Model file for the job. Use its own axes, mm. A direction names the side the tool comes from. Give positions to 0.01 mm unless a question says otherwise; leave off trailing zeros. Loops run counter-clockwise (first coordinate to the right, second up) from the corner with the lowest first, then second, coordinate; pieces in that order, holes last. Notation, with made-up numbers: M -27.75,-7 L 0.25,-7 A21 cw 0.25,18 Z; hole C 33,-40 d9. An arc over 180 degrees is marked long. Answer in a Markdown table with one row per item.
```python
from build123d import *

# Parameters (mm, degrees)
BOSS_EXTRUDE1_DEPTH     = 13
SKETCH6_W               = 6
SKETCH6_H               = 5
BOSS_EXTRUDE4_DEPTH     = 5.6
SKETCH16_W              = 6
SKETCH16_H              = 8
BOSS_EXTRUDE5_DEPTH     = 0.1
CUT_EXTRUDE6_DEPTH      = 4
CUT_EXTRUDE6_DEPTH_BACK = 3.6
SKETCH15_R              = 1.2
CUT_EXTRUDE7_DEPTH      = 8.7202
CUT_EXTRUDE8_START      = -0.2202
SKETCH19_W              = 6
SKETCH19_H              = 8
SKETCH19_R              = 1.2
CUT_EXTRUDE8_DEPTH      = 0.2202
SKETCH12_R              = 1.5
CUT_EXTRUDE5_DEPTH      = 6
CHAMFER1_SIZE           = 0.2
SKETCH20_W              = 5
SKETCH20_H              = 5.5
BOSS_EXTRUDE6_DEPTH     = 0.5
SKETCH21_W              = 5
SKETCH21_H              = 5.5
BOSS_EXTRUDE7_DEPTH     = 0.5
CHAMFER2_SIZE           = 0.2


with BuildPart() as part:
    # Sketch1 → Boss-Extrude1 (new body)
    with BuildSketch(Plane.XY):
        Polygon((3, 3.05), (3, -2.253801214), (2.388188946, -2.95), (-2.388188946, -2.95), (-3, -2.253801214), (-3, 3.05), align=None)
    extrude(amount=BOSS_EXTRUDE1_DEPTH)

    # Sketch6 → Boss-Extrude4 (add)
    with BuildSketch(Plane(origin=(0, 3.05, 0), x_dir=(1, 0, 0), z_dir=(0, 1, 0))):
        with Locations((0, -2.5)):
            Rectangle(SKETCH6_W, SKETCH6_H)
    extrude(amount=BOSS_EXTRUDE4_DEPTH)

    # Sketch16 → Boss-Extrude5 (add)
    with BuildSketch(Plane(origin=(0, 3.05, 0), x_dir=(1, 0, 0), z_dir=(0, 1, 0))):
        with Locations((0, -9)):
            Rectangle(SKETCH16_W, SKETCH16_H)
    extrude(amount=BOSS_EXTRUDE5_DEPTH)

    # Sketch18 → Cut-Extrude6 (cut, two sides: drawn at the far end of the back side and taken through both)
    with BuildSketch(Plane(origin=(0, 0, 0), x_dir=(0, 0, -1), z_dir=(1, 0, 0)).offset(-CUT_EXTRUDE6_DEPTH_BACK)):
        with BuildLine():
            Line((-8.8572, -0.0702), (-12.8572, -0.0702))
            Line((-12.8572, -0.0702), (-13, -0.0702))
            Line((-13, -0.0702), (-13, -0.7))
            Line((-13, -0.7), (-12.8572, -0.7))
            Line((-12.8572, -0.7), (-12.7144, -0.7))
            add(Edge.make_bspline(
                [(-12.7144, -0.7), (-12.5198, -0.7), (-12.43, -0.9509)],
                knots=[0.103448276, 0.103448276, 0.103448276, 0.137931034, 0.137931034, 0.137931034], degree=2))
            add(Edge.make_bspline(
                [(-12.43, -0.9509), (-12.3594, -1.2388), (-12.13, -1.45), (-11.8572, -1.45)],
                knots=[0.137931034, 0.137931034, 0.137931034, 0.137931034, 0.172413793, 0.172413793, 0.172413793, 0.172413793], degree=3))
            add(Edge.make_bspline(
                [(-11.8572, -1.45), (-11.5844, -1.45), (-11.355, -1.2388), (-11.2844, -0.9509)],
                knots=[0.172413793, 0.172413793, 0.172413793, 0.172413793, 0.206896552, 0.206896552, 0.206896552, 0.206896552], degree=3))
            add(Edge.make_bspline(
                [(-11.2844, -0.9509), (-11.1946, -0.7), (-11, -0.7)],
                knots=[0.206896552, 0.206896552, 0.206896552, 0.24137931, 0.24137931, 0.24137931], degree=2))
            Line((-11, -0.7), (-10.8572, -0.7))
            Line((-10.8572, -0.7), (-10.7144, -0.7))
            add(Edge.make_bspline(
                [(-10.7144, -0.7), (-10.5198, -0.7), (-10.43, -0.9509)],
                knots=[0.310344828, 0.310344828, 0.310344828, 0.344827586, 0.344827586, 0.344827586], degree=2))
            add(Edge.make_bspline(
                [(-10.43, -0.9509), (-10.3594, -1.2388), (-10.13, -1.45), (-9.8572, -1.45)],
                knots=[0.344827586, 0.344827586, 0.344827586, 0.344827586, 0.379310345, 0.379310345, 0.379310345, 0.379310345], degree=3))
            add(Edge.make_bspline(
                [(-9.8572, -1.45), (-9.5844, -1.45), (-9.355, -1.2388), (-9.2844, -0.9509)],
                knots=[0.379310345, 0.379310345, 0.379310345, 0.379310345, 0.413793103, 0.413793103, 0.413793103, 0.413793103], degree=3))
            add(Edge.make_bspline(
                [(-9.2844, -0.9509), (-9.1946, -0.7), (-9, -0.7)],
                knots=[0.413793103, 0.413793103, 0.413793103, 0.448275862, 0.448275862, 0.448275862], degree=2))
            Line((-9, -0.7), (-8.8572, -0.7))
            Line((-8.8572, -0.7), (-8.7144, -0.7))
            add(Edge.make_bspline(
                [(-8.7144, -0.7), (-8.5198, -0.7), (-8.43, -0.9509)],
                knots=[0.517241379, 0.517241379, 0.517241379, 0.551724138, 0.551724138, 0.551724138], degree=2))
            add(Edge.make_bspline(
                [(-8.43, -0.9509), (-8.3594, -1.2388), (-8.13, -1.45), (-7.8572, -1.45)],
                knots=[0.551724138, 0.551724138, 0.551724138, 0.551724138, 0.586206897, 0.586206897, 0.586206897, 0.586206897], degree=3))
            add(Edge.make_bspline(
                [(-7.8572, -1.45), (-7.5844, -1.45), (-7.355, -1.2388), (-7.2844, -0.9509)],
                knots=[0.586206897, 0.586206897, 0.586206897, 0.586206897, 0.620689655, 0.620689655, 0.620689655, 0.620689655], degree=3))
            add(Edge.make_bspline(
                [(-7.2844, -0.9509), (-7.1946, -0.7), (-7, -0.7)],
                knots=[0.620689655, 0.620689655, 0.620689655, 0.655172414, 0.655172414, 0.655172414], degree=2))
            Line((-7, -0.7), (-6.8572, -0.7))
            Line((-6.8572, -0.7), (-6.7144, -0.7))
            add(Edge.make_bspline(
                [(-6.7144, -0.7), (-6.5198, -0.7), (-6.43, -0.9509)],
                knots=[0.724137931, 0.724137931, 0.724137931, 0.75862069, 0.75862069, 0.75862069], degree=2))
            add(Edge.make_bspline(
                [(-6.43, -0.9509), (-6.3594, -1.2388), (-6.13, -1.45), (-5.8572, -1.45)],
                knots=[0.75862069, 0.75862069, 0.75862069, 0.75862069, 0.793103448, 0.793103448, 0.793103448, 0.793103448], degree=3))
            add(Edge.make_bspline(
                [(-5.8572, -1.45), (-5.5844, -1.45), (-5.355, -1.2388), (-5.2844, -0.9509)],
                knots=[0.793103448, 0.793103448, 0.793103448, 0.793103448, 0.827586207, 0.827586207, 0.827586207, 0.827586207], degree=3))
            add(Edge.make_bspline(
                [(-5.2844, -0.9509), (-5.1946, -0.7), (-5, -0.7)],
                knots=[0.827586207, 0.827586207, 0.827586207, 0.862068966, 0.862068966, 0.862068966], degree=2))
            Line((-5, -0.7), (-5, -0.0702))
            Line((-5, -0.0702), (-8.8572, -0.0702))
        make_face()
    extrude(amount=CUT_EXTRUDE6_DEPTH + CUT_EXTRUDE6_DEPTH_BACK, mode=Mode.SUBTRACT)

    # Sketch15 → Cut-Extrude7 (cut)
    with BuildSketch(Plane(origin=(0, 8.65, 0), x_dir=(1, 0, 0), z_dir=(0, 1, 0))):
        with Locations(Location((0, -10.8572, 0), (0, 0, 180))):
            Circle(SKETCH15_R)
        with Locations(Location((0, -6.8572, 0), (0, 0, 180))):
            Circle(SKETCH15_R)
    extrude(amount=-CUT_EXTRUDE7_DEPTH, mode=Mode.SUBTRACT)

    # Sketch19 → Cut-Extrude8 (cut)
    with BuildSketch(Plane.XZ.offset(0.0702).offset(CUT_EXTRUDE8_START)):
        with Locations((0, 9)):
            Rectangle(SKETCH19_W, SKETCH19_H)
        with Locations(Location((0, 10.8572, 0), (0, 0, 180))):
            Circle(SKETCH19_R, mode=Mode.SUBTRACT)
        with Locations(Location((0, 6.8572, 0), (0, 0, 180))):
            Circle(SKETCH19_R, mode=Mode.SUBTRACT)
    extrude(amount=CUT_EXTRUDE8_DEPTH, mode=Mode.SUBTRACT)

    # Sketch12 → Cut-Extrude5 (cut)
    with BuildSketch(Plane.XY.offset(5)):
        with Locations((0, 5.9)):
            Circle(SKETCH12_R)
    extrude(amount=-CUT_EXTRUDE5_DEPTH, mode=Mode.SUBTRACT)

    # Chamfer1
    chamfer1_edges = [part.edges().sort_by_distance(p)[0] for p in [
        (-2.694094473, -2.601900607, 13),
        (0, -2.95, 13),
        (2.694094473, -2.601900607, 13),
        (3, 1.65, 13),
        (3, -1.476900607, 13),
        (-3, -1.476900607, 13),
        (-3, 1.65, 13),
    ]]
    chamfer(chamfer1_edges, length=CHAMFER1_SIZE)

    # Sketch20 → Boss-Extrude6 (add)
    with BuildSketch(Plane(origin=(3, 0, 0), x_dir=(0, 0, -1), z_dir=(1, 0, 0))):
        with Locations((-2.5, 5.9)):
            Rectangle(SKETCH20_W, SKETCH20_H)
    extrude(amount=BOSS_EXTRUDE6_DEPTH)

    # Sketch21 → Boss-Extrude7 (add)
    with BuildSketch(Plane.ZY.offset(3)):
        with Locations((2.5, 5.9)):
            Rectangle(SKETCH21_W, SKETCH21_H)
    extrude(amount=BOSS_EXTRUDE7_DEPTH)

    # Chamfer2
    chamfer2_edges = [part.edges().sort_by_distance(p)[0] for p in [
        (3.5, 5.9, 5),
        (-3.5, 5.9, 5),
    ]]
    chamfer(chamfer2_edges, length=CHAMFER2_SIZE)


solid = part.part
```
(1) Mould opens along Y. For faces 4 (the flat face through (0, 8.65, 2)), 5 (the flat face through (-3, 0.4, 6.5)), 6 (the flat face through (0, -2.95, 6)), 7 (the cylindrical face through (-0.195, 7.387, 2.535)) say: pulls with the +Y half, pulls with the -Y half, needs draft (parallel to the pull), parting line crosses it, or undercut.
Established:
| item | result |
|---|---|
| face 4 | pulls with the +Y half |
| face 5 | needs draft |
| face 6 | pulls with the -Y half |
| face 7 | undercut |
(2) Saw through at C-C, the plane x = 0. Count the separate pieces of the cut face and the enclosed holes in it, and give its area (3 significant figures).
Established:
| item | result |
|---|---|
| separate pieces | 4 |
| enclosed holes | 0 |
| area | 67.6 mm2 |
(3) Flat gauge pins, fed straight in: P1, Ø4, axis at x = 0, y = 5.9, coming from the +Z side; P2, Ø2, axis at x = 1, y = 3, coming from the -Z side; P3, Ø3, axis at y = 1.5, z = 8.5, coming from the +X side; P4, Ø1, axis at x = -1.5, z = 10.5, coming from the +Y side. Where does each tip first touch, or does it go through?
Established:
| item | result |
|---|---|
| P1 | stops at z = 5 |
| P2 | stops at z = 0 |
| P3 | stops at x = 3 |
| P4 | stops at y = 3.15 |
(4) Saw through at B-B, the plane z = 1.5. Give the cut face in (x, y).
Established:
| item | result |
|---|---|
| outline | M -3.5,3.15 L -3,3.15 L -3,-2.25 L -2.39,-2.95 L 2.39,-2.95 L 3,-2.25 L 3,3.15 L 3.5,3.15 L 3.5,8.65 L -3.5,8.65 Z; hole C 0,5.9 d3 |
(5) Which spindle directions (+Z, -Z, +X, -X, +Y, -Y) get a long thin tool onto all of the face, cutting with end or side? Do faces 1 (the cylindrical face through (0.26, 1.671, 5.686)), 2 (the flat face through (0, 3.15, 9)), 3 (the flat face through (0, 0.15, 9)). Say none if no direction does.
Established:
| item | result |
|---|---|
| face 1 | +Y |
| face 2 | +Z, +X, -X, +Y |
| face 3 | +Z, +X, -X |
(6) Saw through at A-A, the plane y = 5.9. Give the cut face in (x, z), and give its area (3 significant figures).
Established:
| item | result |
|---|---|
| outline | M -3.5,0 L -1.5,0 L -1.5,5 L -3.3,5 L -3.5,4.8 Z; M 1.5,0 L 3.5,0 L 3.5,4.8 L 3.3,5 L 1.5,5 Z |
| area | 20.0 mm2 |
(7) Wall check: L1, parallel to Z at x = 0, y = 2.2; L2, parallel to Z at x = -0.75, y = 1.75; L3, parallel to Y at x = 0, z = 1.8. Give the ranges that are in metal, low to high.
Established:
| item | result |
|---|---|
| L1 | z = 0 to 5.66, 8.06 to 9.66, 12.06 to 13 |
| L2 | z = 0 to 5.92, 7.79 to 9.92, 11.79 to 13 |
| L3 | y = -2.95 to 4.4, 7.4 to 8.65 |
